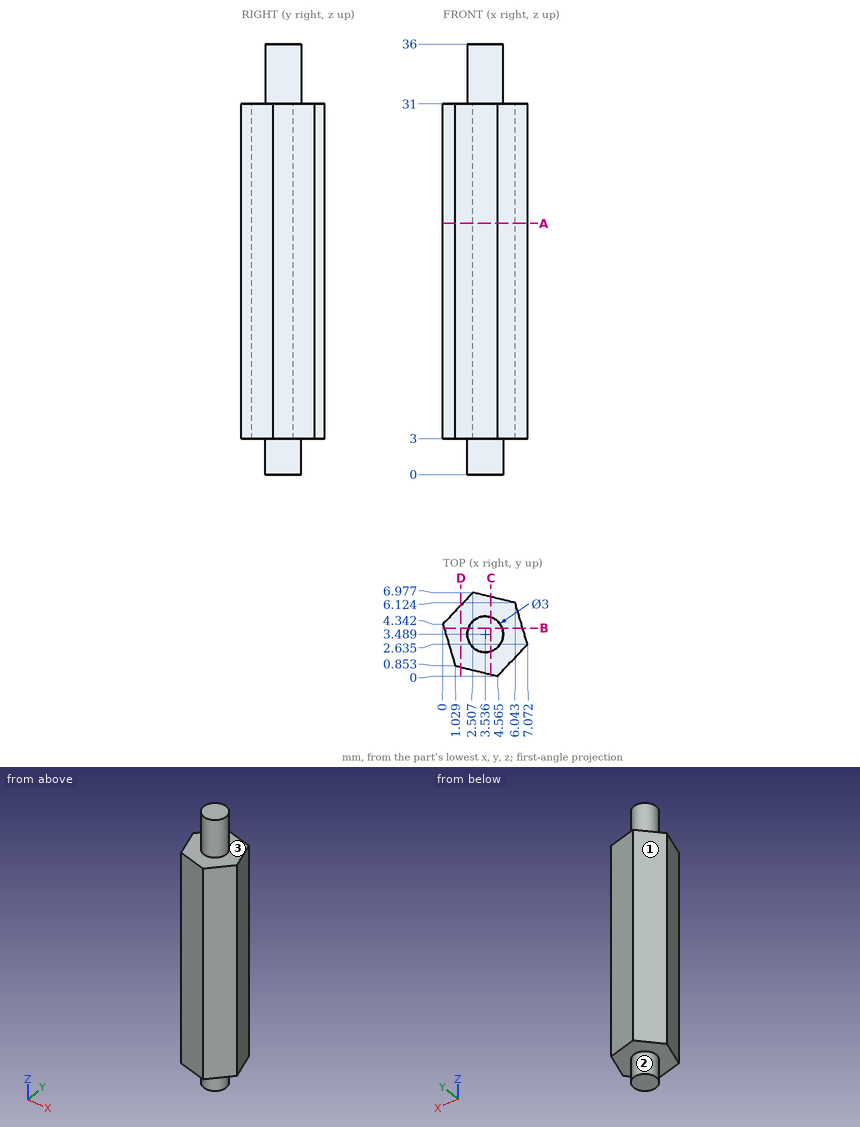
Can you work these out from the drawing? Everything is in mm from the part's minimum corner. A direction names the side the tool comes from. Give positions to 0.01 mm unless a question says otherwise; leave off trailing zeros. Write each loop counter-clockwise with the first axis right and the second up, starting at its lowest first coordinate (ties: lowest second). Pieces come first, ordered by that corner, then holes. Notation, with made-up numbers: M 31,57 L 61,57 A15 cw 61,86 Z; hole C 46.25,49.5 d11. An arc over 180 degrees is marked long. Answer in a Markdown table with one row per item. Add a question column.
Item 1: Imagine slicing it at D-D, the plane x = 1.5. Write out the boundary of the cut face in (y, z).
Item 2: On a 3-axis mill with a long thin cutter (end or side, diameter ignored), from which of +Z, -Z, +X, -X, +Y, -Y can I reach the whole of each face in a straight line? I mean the marked faces 1, 2 and 3. Say none if no direction works.
Item 3: Imagine slicing it at B-B, the plane y = 4. Write out the boundary of the cut face in (x, z) (1 decimal).
Item 4: For pin 1 Ø1 at (y, z) = (5, 13) entering from -X, with a flat end and sliding along its axis, tell me the tip position at first contact or that it passes through.
Item 5: Imagine slicing it at A-A, the plane z = 21. Write out the boundary of the cut face in (x, y) (1 decimal), plus the area to 3 significant figures.
Item 6: Please list where these lines run through material, in increasing order: L1, parallel to Z at x = 2.5, y = 6; L2, parallel to X at y = 5.5, z = 30 (1 decimal); L3, parallel to Y at x = 3, z = 19.
Item 7: Imagine slicing it at C-C, the plane x = 4. Write out the boundary of the cut face in (y, z) (1 decimal), plus the area to 3 significant figures.
Evaluation:
| question | item | result |
|---|---|---|
| 1 | outline | M 0.74,3 L 5.92,3 L 5.92,31 L 0.74,31 Z |
| 2 | face 1 | +Z, -Z, -X, +Y |
| 2 | face 2 | -Z |
| 2 | face 3 | +Z |
| 3 | outline | M 0.1,3 L 2.1,3 L 2.1,0 L 4.9,0 L 4.9,3 L 6.7,3 L 6.7,31 L 4.9,31 L 4.9,36 L 2.1,36 L 2.1,31 L 0.1,31 Z |
| 4 | pin 1 | stops at x = 0.15 |
| 5 | outline | M 0,4.3 L 1,0.9 L 4.6,0 L 7.1,2.6 L 6,6.1 L 2.5,7 Z |
| 5 | area | 34.4 mm² |
| 6 | L1 | z = 3 to 31 |
| 6 | L2 | x = 1.1 to 6.2 |
| 6 | L3 | y = 0.38 to 6.86 |
| 7 | outline | M 0.1,3 L 2.1,3 L 2.1,0 L 4.9,0 L 4.9,3 L 6.6,3 L 6.6,31 L 4.9,31 L 4.9,36 L 2.1,36 L 2.1,31 L 0.1,31 Z |
| 7 | area | 204 mm² |
